Work out the finished part from the listing and answer in its coordinate system (mm). Face numbers are marked on the shaded views. A direction names the side the tool comes from. Coordinates: 2 decimals unless noted, no trailing zeros. Order: outer loops, then holes, each group sorted by start corner. A loop starts at its lowest first (then second) coordinate and runs counter-clockwise, first axis right, second up. Notation, with made-up numbers: (-33, 11.5) -> (4, 11.5) arc R29 cw to (4, 49.5) -> close; hole circle Ø7 at (-11, 0.25). An arc over 180 degrees is marked (long way). Write item = value, one per line. Start each with the question number.
Q1. The part is cut by section B-B, the plane y = -4.5. Determine the outline of the cut face in (x, z), plus the area to 3 significant figures.
Q2. Flat-ended cylindrical pins translate along their axes: pin 1 (8 mm diameter, centred on y = -3.5, z = 4.5, fed in from +X); pin 2 (1.5 mm diameter, centred on x = 17.5, y = -5.5, fed in from -Z); pin 3 (5 mm diameter, centred on y = -7.5, z = 5.5, fed in from +X). Find the tip coordinate at first contact, or state that the pin passes through.
Q3. The part is cut by section A-A, the plane z = 1.5. Determine the outline of the cut face in (x, y).
Q4. The part is cut by section D-D, the plane y = -1.5. Determine the outline of the cut face in (x, z), plus the area to 4 significant figures.
Q5. Which of the six approach directions +Z, -Z, +X, -X, +Y, -Y give full straight-line access (tool end or side, diameter ignored) to the marked faces 1 and 2?
Q6. The part is cut by section C-C, the plane z = 11. Determine the outline of the cut face in (x, y), plus the area to 3 significant figures.
Q7. For a pull along X with two mould halves and no side action, classify the marked faces 3, 4 and 5 as +X half, -X half, draft (parallel to the pull), parting line (faces both ways), or undercut.
Q8. Straight lines are drawn through the part: L1, parallel to Y at x = 26.25, z = 2; L2, parallel to X at y = -9.5, z = 10.5; L3, parallel to Z at x = 7.5, y = -6. For each, find the intervals that lie inside material, in ascending order. Write a range as from..to.
```python
from build123d import *

# Parameters (mm, degrees)
F1_DEPTH = 15
F2_W     = 10
F2_H     = 10
F3_DEPTH = 25


with BuildPart() as f1:
    # F0 (on Front) → F1 (new body)
    with BuildSketch(Plane.XZ):
        Polygon((0, 20), (0, 0), (5, 0), (5, 2.5), (20, 2.5), (20, 0), (30, 0), (30, 7.5), (10, 20), align=None)
    extrude(amount=F1_DEPTH)

    # F2 (on face) → F3 (cut)
    with BuildSketch(Plane(origin=(0, 0, 0), x_dir=(1, 0, 0), z_dir=(0, 0, -1))):
        with Locations((25, 7.5)):
            Rectangle(F2_W, F2_H)
    extrude(amount=-F3_DEPTH, mode=Mode.SUBTRACT)


solid = f1.part
```
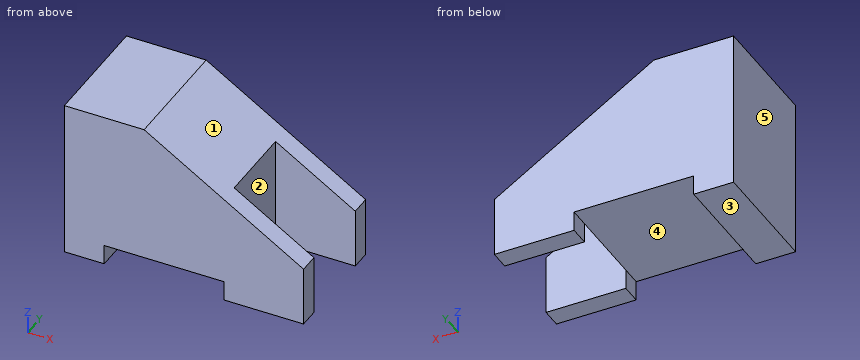
Model answer:
q1.outline = (0, 0) -> (5, 0) -> (5, 2.5) -> (20, 2.5) -> (20, 13.75) -> (10, 20) -> (0, 20) -> close
q1.area = 331 mm2
q2.pin_1 = 30
q2.pin_2 = 2.5
q2.pin_3 = 20
q3.outline = (0, -15) -> (5, -15) -> (5, 0) -> (0, 0) -> close; (20, -15) -> (30, -15) -> (30, -12.5) -> (20, -12.5) -> close; (20, -2.5) -> (30, -2.5) -> (30, 0) -> (20, 0) -> close
q4.outline = (0, 0) -> (5, 0) -> (5, 2.5) -> (20, 2.5) -> (20, 0) -> (30, 0) -> (30, 7.5) -> (10, 20) -> (0, 20) -> close
q4.area = 437.5 mm2
q5.face_1 = +Z, +X, +Y, -Y
q5.face_2 = +Z, -Z, +X
q6.outline = (0, -15) -> (24.4, -15) -> (24.4, -12.5) -> (20, -12.5) -> (20, -2.5) -> (24.4, -2.5) -> (24.4, 0) -> (0, 0) -> close
q6.area = 322 mm2
q7.face_3 = draft
q7.face_4 = undercut
q7.face_5 = -X half
q8.L1 = -15..-12.5, -2.5..0
q8.L2 = 0..20
q8.L3 = 2.5..20
